Design review of the part built by this model. Coordinates are the model's own, in mm. A direction names the side the tool comes from. Coordinates: 2 decimals unless noted, no trailing zeros. Write each loop counter-clockwise with the first axis right and the second up, starting at its lowest first coordinate (ties: lowest second). Pieces come first, ordered by that corner, then holes. Notation, with made-up numbers: M -26.75,-4.5 L -3.75,-4.5 A20 cw -3.75,14.5 Z; hole C -5.5,81.25 d8. An arc over 180 degrees is marked long. One line per question, with ' | ' between items.
from build123d import *

# Parameters (mm, degrees)
SKETCH1_W           = 67
SKETCH1_H           = 50
BOSS_EXTRUDE1_DEPTH = 70
SKETCH3_W           = 29
SKETCH3_H           = 3.3
CUT_EXTRUDE1_DEPTH  = 67
SKETCH4_R           = 20
CUT_EXTRUDE2_DEPTH  = 1.5
CUT_EXTRUDE3_START  = -1.5
SKETCH5_R           = 20
CUT_EXTRUDE3_DEPTH  = 1.5
SKETCH7_R           = 3.15
CUT_EXTRUDE4_DEPTH  = 12.5
CUT_EXTRUDE5_DEPTH  = 1.5


with BuildPart() as part:
    # Sketch1 → Boss-Extrude1 (new body)
    with BuildSketch(Plane(origin=(0, 0, 0), x_dir=(1, 0, 0), z_dir=(0, 1, 0))):
        Rectangle(SKETCH1_W, SKETCH1_H)
    extrude(amount=BOSS_EXTRUDE1_DEPTH)

    # Sketch3 → Cut-Extrude1 (cut)
    with BuildSketch(Plane(origin=(33.5, 0, 0), x_dir=(0, 0, -1), z_dir=(1, 0, 0))):
        with Locations((10.5, 55.85)):
            Rectangle(SKETCH3_W, SKETCH3_H)
        with BuildLine():
            Line((25, 36.5), (25, 17.5))
            Line((25, 17.5), (18.454482672, 17.5))
            ThreePointArc((18.454482672, 17.5), (-17, 27), (18.454482672, 36.5))
            Line((18.454482672, 36.5), (25, 36.5))
        make_face()
    extrude(amount=-CUT_EXTRUDE1_DEPTH, mode=Mode.SUBTRACT)

    # Sketch4 → Cut-Extrude2 (cut)
    with BuildSketch(Plane(origin=(21, 0, 0), x_dir=(0, 0, -1), z_dir=(1, 0, 0))):
        with Locations((2, 27)):
            Circle(SKETCH4_R)
    extrude(amount=CUT_EXTRUDE2_DEPTH, mode=Mode.SUBTRACT)

    # Sketch5 → Cut-Extrude3 (cut)
    with BuildSketch(Plane(origin=(-21, 0, 0), x_dir=(0, 0, -1), z_dir=(1, 0, 0)).offset(CUT_EXTRUDE3_START)):
        with Locations((2, 27)):
            Circle(SKETCH5_R)
    extrude(amount=CUT_EXTRUDE3_DEPTH, mode=Mode.SUBTRACT)

    # Sketch7 → Cut-Extrude4 (cut)
    with BuildSketch(Plane(origin=(0, 70, 0), x_dir=(1, 0, 0), z_dir=(0, 1, 0))):
        with Locations(Location((0, 16.7, 0), (0, 0, 270))):
            Circle(SKETCH7_R)
    extrude(amount=-CUT_EXTRUDE4_DEPTH, mode=Mode.SUBTRACT)

    # Sketch9 → Cut-Extrude5 (cut)
    with BuildSketch(Plane.XY.offset(25)):
        Polygon((-33.5, 0), (-33.5, 4.8), (-6.317148544, 35), (-33.5, 65.2), (-33.5, 70), (-25.186156124, 70), (0, 42.018317645), (25.186156124, 70), (33.5, 70), (33.5, 65.2), (6.317148544, 35), (33.5, 4.8), (33.5, 0), (25.186156124, 0), (0, 27.981682355), (-25.186156124, 0), align=None)
    extrude(amount=-CUT_EXTRUDE5_DEPTH, mode=Mode.SUBTRACT)


solid = part.part
1. Take a section at D-D (y = 25). Write out the cut boundary in (x, z).
Answer sheet:
outline: M -33.5,16.89 L -22.5,16.89 L -22.5,17.9 L -21,17.9 L -21,16.89 L 21,16.89 L 21,17.9 L 22.5,17.9 L 22.5,16.89 L 33.5,16.89 L 33.5,25 L 15.32,25 L 15.32,23.5 L 2.68,23.5 L 2.68,25 L -2.68,25 L -2.68,23.5 L -15.32,23.5 L -15.32,25 L -33.5,25 Z
2. Take a section at A-A (z = -16.7). Count the separate pieces of the cut face and the enclosed holes in it, then the cut area to 3 significant figures.
Answer sheet:
separate pieces: 4 | enclosed holes: 0 | area: 2,770 mm^2
3. Insertion check: pin 1 Ø8.5 at (x, z) = (-8.5, -12) entering from -Y; pin 2 Ø1 at (x, y) = (4, 25.5) entering from +Z. Each pin has a flat end and moves straight along its axis. Give the tip position at first contact, or say it passes through.
Answer sheet:
pin 1: y = 0 | pin 2: z = 23.5
4. To check wall thickness, follow line 1 along Y through (x, z) = (28, -2); line 2 along Y through (x, z) = (21.5, -2); line 3 along Z through (x, y) = (21.35, 27). State the ranges of each line that lie inside material, in increasing order. Write a range as [from, to].
Answer sheet:
line 1: [0, 8], [46, 54.2], [57.5, 70] | line 2: [0, 7], [47, 54.2], [57.5, 70] | line 3: [18, 25]
5. Take a section at C-C (x = 9.5). Write out the cut boundary in (y, z).
Answer sheet:
outline: M 0,-25 L 17.5,-25 L 17.5,-18.45 A19 cw long 36.5,-18.45 L 36.5,-25 L 54.2,-25 L 54.2,4 L 57.5,4 L 57.5,-25 L 70,-25 L 70,25 L 52.57,25 L 52.57,23.5 L 38.54,23.5 L 38.54,25 L 31.46,25 L 31.46,23.5 L 17.43,23.5 L 17.43,25 L 0,25 Z
6. Tool access review of faces 4 (the face through (0, 36.5, -22)), 5 (the face through (-22.5, 27.1, 17.4)), 6 (the face through (-12.769, 56.205, 24.26)): name each direction out of +Z, -Z, +X, -X, +Y, -Y from which nothing blocks a thin tool from reaching the whole face with its end or side.
Answer sheet:
face 4: -Z, +X, -X | face 5: none | face 6: +Z
7. Draft analysis for pull direction Y (two halves, no side actions). For faces 1 (the face through (0, 0, 0)), 2 (the face through (21, 27.1, 17.4)), 3 (the face through (0, 59, 25)), state which applies: pulls with the +Y half, pulls with the -Y half, needs draft (parallel to the pull), parting line crosses it, or undercut.
Answer sheet:
face 1: pulls with the -Y half | face 2: undercut | face 3: needs draft
8. Take a section at B-B (z = -7). Write out the cut boundary in (x, y), then the cut area to 3 significant figures.
Answer sheet:
outline: M -33.5,0 L 33.5,0 L 33.5,8.67 L 22.5,8.67 L 22.5,7.64 L 21,7.64 L 21,8.67 L -21,8.67 L -21,7.64 L -22.5,7.64 L -22.5,8.67 L -33.5,8.67 Z; M -33.5,45.33 L -22.5,45.33 L -22.5,46.36 L -21,46.36 L -21,45.33 L 21,45.33 L 21,46.36 L 22.5,46.36 L 22.5,45.33 L 33.5,45.33 L 33.5,54.2 L -33.5,54.2 Z; M -33.5,57.5 L 33.5,57.5 L 33.5,70 L -33.5,70 Z | area: 2,010 mm^2
